```python
from build123d import *

# Parameters (mm, degrees)
SKETCH1_R           = 19
SKETCH1_R_2         = 1.75
SKETCH1_W           = 30
SKETCH1_H           = 3
SKETCH1_W_2         = 10
BOSS_EXTRUDE3_DEPTH = 3


with BuildPart() as part:
    # Sketch1 → Boss-Extrude3 (new body)
    with BuildSketch(Plane.XY):
        with BuildLine():
            Line((-47.5, 30), (47.5, 30))
            Line((47.5, 30), (47.5, 24))
            Line((47.5, 24), (50.5, 24))
            Line((50.5, 24), (50.5, 14))
            Line((50.5, 14), (47.5, 14))
            Line((47.5, 14), (47.5, 6.5))
            Line((47.5, 6.5), (45, 6.5))
            Line((45, 6.5), (45, 8))
            Line((45, 8), (42, 8))
            Line((42, 8), (42, 6.5))
            Line((42, 6.5), (38.5, 6.5))
            Line((38.5, 6.5), (38.5, 3.5))
            Line((38.5, 3.5), (42, 3.5))
            Line((42, 3.5), (42, 2))
            Line((42, 2), (45, 2))
            Line((45, 2), (45, 3.5))
            Line((45, 3.5), (47.5, 3.5))
            Line((47.5, 3.5), (47.5, -5))
            Line((47.5, -5), (67.5, -5))
            ThreePointArc((67.5, -5), (74.571067812, -7.928932188), (77.5, -15))
            Line((77.5, -15), (77.5, -30))
            Line((77.5, -30), (77.5, -40))
            Line((77.5, -40), (-47.5, -40))
            Line((-47.5, -40), (-47.5, -30))
            Line((-47.5, -30), (-47.5, -24))
            Line((-47.5, -24), (-50.5, -24))
            Line((-50.5, -24), (-50.5, -14))
            Line((-50.5, -14), (-47.5, -14))
            Line((-47.5, -14), (-47.5, -1.5))
            Line((-47.5, -1.5), (-45, -1.5))
            Line((-45, -1.5), (-45, -3))
            Line((-45, -3), (-42, -3))
            Line((-42, -3), (-42, -1.5))
            Line((-42, -1.5), (-38.5, -1.5))
            Line((-38.5, -1.5), (-38.5, 1.5))
            Line((-38.5, 1.5), (-42, 1.5))
            Line((-42, 1.5), (-42, 3))
            Line((-42, 3), (-45, 3))
            Line((-45, 3), (-45, 1.5))
            Line((-45, 1.5), (-47.5, 1.5))
            Line((-47.5, 1.5), (-47.5, 14))
            Line((-47.5, 14), (-50.5, 14))
            Line((-50.5, 14), (-50.5, 24))
            Line((-50.5, 24), (-47.5, 24))
            Line((-47.5, 24), (-47.5, 30))
        make_face()
        Circle(SKETCH1_R, mode=Mode.SUBTRACT)
        with Locations((-26, -26.5)):
            Circle(SKETCH1_R_2, mode=Mode.SUBTRACT)
        with Locations((34, -26.5)):
            Circle(SKETCH1_R_2, mode=Mode.SUBTRACT)
        with Locations((34, -34.5)):
            Circle(SKETCH1_R_2, mode=Mode.SUBTRACT)
        with Locations((57.5, -26.5)):
            Rectangle(SKETCH1_W, SKETCH1_H, mode=Mode.SUBTRACT)
        with Locations((-32.5, 16.5)):
            Rectangle(SKETCH1_W_2, SKETCH1_H, mode=Mode.SUBTRACT)
        with Locations((32.5, 16.5)):
            Rectangle(SKETCH1_W_2, SKETCH1_H, mode=Mode.SUBTRACT)
        with Locations((57.5, -34.5)):
            Rectangle(SKETCH1_W, SKETCH1_H, mode=Mode.SUBTRACT)
    extrude(amount=BOSS_EXTRUDE3_DEPTH)


solid = part.part
```
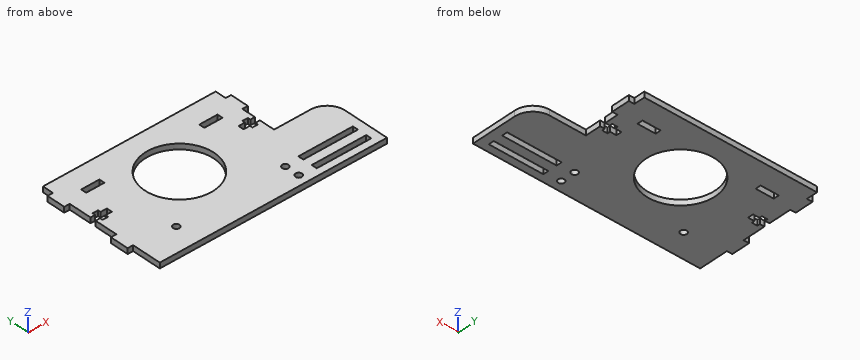
Design review of the part built by this model. Coordinates are the model's own, in mm. Give positions to 0.01 mm unless a question says otherwise; leave off trailing zeros. Loops run counter-clockwise (first coordinate to the right, second up) from the corner with the lowest first, then second, coordinate; pieces in that order, holes last. Notation, with made-up numbers: (14.25, -39.75) -> (59.25, -39.75) arc R25 cw to (59.25, -14.75) -> close; hole circle Ø5 at (84.25, -10.5). An arc over 180 degrees is marked (long way). One line per item, written item: value.
Q1. We need section B-B on y = -34.5. Give the boundary of the cut face in (x, z), and give its area (4 significant figures).
Numbers:
outline: (-47.5, 0) -> (32.25, 0) -> (32.25, 3) -> (-47.5, 3) -> close; (35.75, 0) -> (42.5, 0) -> (42.5, 3) -> (35.75, 3) -> close; (72.5, 0) -> (77.5, 0) -> (77.5, 3) -> (72.5, 3) -> close
area: 274.5 mm^2
Q2. For pin 1 Ø1.2 at (y, z) = (7, 1) entering from +X; pin 2 Ø8 at (x, y) = (-32, 20.5) entering from -Z; pin 3 Ø3 at (x, y) = (-26, -26.5) entering from +Z; pin 4 Ø1.6 at (y, z) = (-2.5, 1) entering from -X, all flat-tipped, find the tip position at first contact; note any pin that passes through.
Numbers:
pin 1: stops at x = 47.5
pin 2: stops at z = 0
pin 3: passes through
pin 4: stops at x = -47.5
Q3. We need section D-D on y = 0. Give the boundary of the cut face in (x, z).
Numbers:
outline: (-38.5, 0) -> (-19, 0) -> (-19, 3) -> (-38.5, 3) -> close; (19, 0) -> (47.5, 0) -> (47.5, 3) -> (19, 3) -> close
Q4. We need section A-A on x = 0. Give the boundary of the cut face in (y, z), and give its area (3 significant figures).
Numbers:
outline: (-40, 0) -> (-19, 0) -> (-19, 3) -> (-40, 3) -> close; (19, 0) -> (30, 0) -> (30, 3) -> (19, 3) -> close
area: 96.0 mm^2
Q5. For L1, parallel to Y at x = 34, z = 1.1; L2, parallel to Y at x = 66, z = 1.85; L3, parallel to X at y = -27, z = 2.75, list the stretches that pass through material, from the lowest coordinate up.
Numbers:
L1: y = -40 to -36.25, -32.75 to -28.25, -24.75 to 15, 18 to 30
L2: y = -40 to -36, -33 to -28, -25 to -5
L3: x = -47.5 to -27.68, -24.32 to 32.32, 35.68 to 42.5, 72.5 to 77.5
Q6. We need section C-C on x = 34. Give the boundary of the cut face in (y, z).
Numbers:
outline: (-40, 0) -> (-36.25, 0) -> (-36.25, 3) -> (-40, 3) -> close; (-32.75, 0) -> (-28.25, 0) -> (-28.25, 3) -> (-32.75, 3) -> close; (-24.75, 0) -> (15, 0) -> (15, 3) -> (-24.75, 3) -> close; (18, 0) -> (30, 0) -> (30, 3) -> (18, 3) -> close
